Part print with two shaded views. Sizes in mm from the minimum x, y, z corner. A direction names the side the tool comes from. Round coordinates to 2 decimals unless told otherwise and drop trailing zeros. Write each loop counter-clockwise with the first axis right and the second up, starting at its lowest first coordinate (ties: lowest second). Pieces come first, ordered by that corner, then holes. Notation, with made-up numbers: (84.5, -0.5) -> (134.5, -0.5) arc R15 cw to (134.5, 6.5) -> close; hole circle Ø3 at (-8.5, 10). An arc over 180 degrees is marked (long way). Return JSON: item names as keys, results as strings. Group by question number.
(1) Saw through at A-A (z = 28.5). List the corners of the cut face in (x, y), plus the area to 3 significant figures.
(2) Saw through at C-C (x = 7.25). List the corners of the cut face in (y, z), plus the area to 3 significant figures.
(3) Saw through at D-D (y = 6.5). List the corners of the cut face in (x, z).
(4) Saw through at B-B (z = 15). List the corners of the cut face in (x, y), plus the area to 3 significant figures.
(5) Tool access for the marked faces 1 and 2: list every direction of +Z, -Z, +X, -X, +Y, -Y with a clear straight run to the whole face (end or side of a thin tool).
(6) Mould opens along Y. For the marked faces 3, 4 and 5 say: +Y half, -Y half, draft (parallel to the pull), parting line (faces both ways), or undercut.
(7) Drop flat-ended pins along their axis: pin 1 Ø2 at (x, z) = (5.5, 22.5) entering from -Y; pin 2 Ø3 at (x, y) = (4, 4) entering from -Z; pin 3 Ø2 at (y, z) = (1, 4) entering from -X; pin 4 Ø3 at (x, y) = (3, 3) entering from -Z. Give the stop position or say it passes through.
(8) Drill centre lines: L1, parallel to Y at x = 4, z = 2.25; L2, parallel to Y at x = 3.25, z = 30 (1 decimal); L3, parallel to X at y = 3, z = 7. Where is each one in solid material? Low to high. Write a range as from..to.
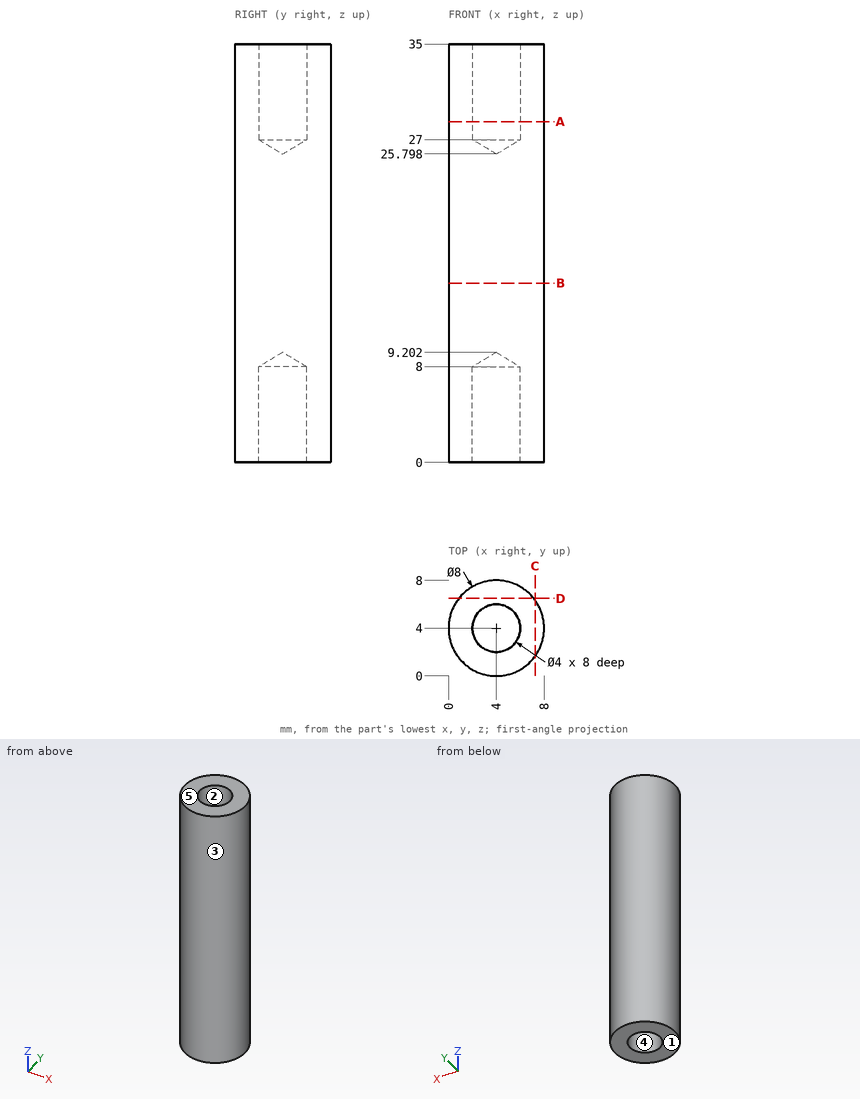
Computed values:
{
 "1": {"outline": "circle Ø8 at (4, 4); hole circle Ø4 at (4, 4)", "area": "37.7 mm2"},
 "2": {"outline": "(1.67, 0) -> (6.33, 0) -> (6.33, 35) -> (1.67, 35) -> close", "area": "163 mm2"},
 "3": {"outline": "(0.88, 0) -> (7.12, 0) -> (7.12, 35) -> (0.88, 35) -> close"},
 "4": {"outline": "circle Ø8 at (4, 4)", "area": "50.3 mm2"},
 "5": {"face 1": "-Z, +X, -X, +Y, -Y", "face 2": "+Z"},
 "6": {"face 3": "parting line", "face 4": "undercut", "face 5": "draft"},
 "7": {"pin 1": "y = 0.03", "pin 2": "z = 8.3", "pin 3": "x = 0.54", "pin 4": "z = 0"},
 "8": {"L1": "0..2, 6..8", "L2": "0.1..2.1, 5.9..7.9", "L3": "0.13..2.27, 5.73..7.87"}
}
